The model under review builds one solid part; all positions refer to its coordinate system, in mm. Face numbers are marked on the shaded views. A direction names the side the tool comes from. Give positions to 0.01 mm unless a question says otherwise; leave off trailing zeros. Order: outer loops, then holes, each group sorted by start corner. A loop starts at its lowest first (then second) coordinate and runs counter-clockwise, first axis right, second up.
```python
from build123d import *

# Parameters (mm, degrees)
F0_R     = 32.4890265079
F0_R_2   = 26.7459939795
F1_DEPTH = 50.8
F2_DEPTH = 25.4
F3_W     = 12.6311182976
F3_H     = 77.5911509991
F4_DEPTH = 88.9
F5_DEPTH = 1.7660884187


with BuildPart() as f1:
    # F0 (on Top) → F1 (new body)
    with BuildSketch(Plane.XY):
        Circle(F0_R)
        Circle(F0_R_2, mode=Mode.SUBTRACT)
    extrude(amount=F1_DEPTH)

    # F2 (add): a face of the model
    f2_faces = [f1.faces().sort_by_distance(p)[0] for p in [
        (-31.5700980696, 0, 0),
    ]]
    extrude(f2_faces, amount=F2_DEPTH)

    # F3 (on Front) → F4 (join)
    with BuildSketch(Plane.XZ):
        with Locations((0, 11.1875087023)):
            Rectangle(F3_W, F3_H)
    extrude(amount=F4_DEPTH)

    # F5 (add): a face of the model
    f5_faces = [f1.faces().sort_by_distance(p)[0] for p in [
        (0, -60.5913176327, 49.9830842018),
    ]]
    extrude(f5_faces, amount=F5_DEPTH)


solid = f1.part
```
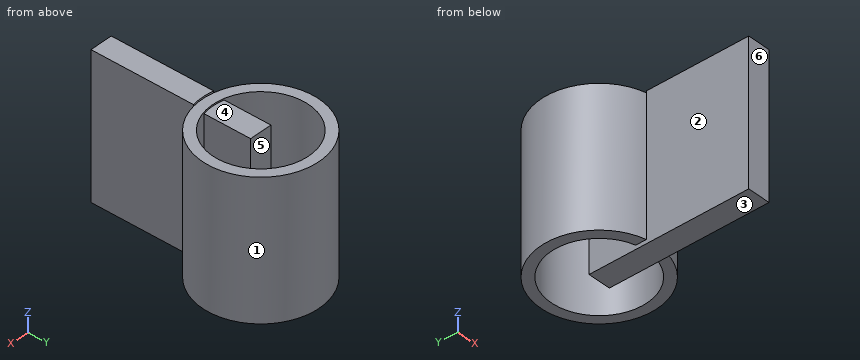
1. Take a section at B-B (y = 16). Write out the cut boundary in (x, z), and give its area (3 significant figures).
2. Draft analysis for pull direction Y (two halves, no side actions). For the marked faces 1, 2, 3 and 4, state which applies: pulls with the +Y half, pulls with the -Y half, needs draft (parallel to the pull), parting line crosses it, or undercut.
3. For the marked faces 5 and 6, list the 3-axis set-ups (+Z, -Z, +X, -X, +Y, -Y) from which the entire face can be reached by the end or side of a thin tool; tool diameter is ignored.
4. Take a section at D-D (z = 39.5). Write out the cut boundary in (x, y), and give its area (3 significant figures).
5. To check wall thickness, follow line 1 (X direction, y = -7, z = 12); line 2 (Y direction, x = 0, z = 20); line 3 (X direction, y = -62, z = -13.5). State the ranges of each line that lie inside material, in increasing order.
6. Insertion check: pin 1 (1 mm diameter, centred on x = 13, z = 14.5, fed in from +Y); pin 2 (10 mm diameter, centred on x = -10, y = -7, fed in from +Z); pin 3 (2 mm diameter, centred on x = -6, z = 19.5, fed in from +Y). Each pin has a flat end and moves straight along its axis. Give the tip position at first contact, or say it passes through.
7. Take a section at A-A (x = 0). Write out the cut boundary in (y, z), and give its area (3 significant figures).
8. Take a section at C-C (y = -10.5). Write out the cut boundary in (x, z), and give its area (3 significant figures).
Answer:
1. outline: (-28.28, -25.4) - (-21.43, -25.4) - (-21.43, 50.8) - (-28.28, 50.8) - close; (21.43, -25.4) - (28.28, -25.4) - (28.28, 50.8) - (21.43, 50.8) - close
1. area: 1,040 mm2
2. face 1: parting line crosses it
2. face 2: undercut
2. face 3: needs draft
2. face 4: undercut
3. face 5: +Z, -Z
3. face 6: +Z, -Z, +X, -X, -Y
4. outline: (-6.32, -88.9) - (6.32, -88.9) - (6.32, -31.87) arc R32.49 ccw (long way) to (-6.32, -31.87) - close; hole (-6.32, -25.99) - (-6.32, 0) - (6.32, 0) - (6.32, -25.99) arc R26.75 ccw (long way) to start
4. area: 2,120 mm2
5. line 1: x = -31.73 to -25.81, -6.32 to 6.32, 25.81 to 31.73
5. line 2: y = -88.9 to 0, 26.75 to 32.49
5. line 3: x = -6.32 to 6.32
6. pin 1: stops at y = 29.99
6. pin 2: stops at z = 49.98
6. pin 3: stops at y = 32.1
7. outline: (-88.9, -27.61) - (0, -27.61) - (0, 49.98) - (-26.75, 49.98) - (-26.75, 50.8) - (-32.49, 50.8) - (-32.49, 51.75) - (-88.9, 51.75) - close; (26.75, -25.4) - (32.49, -25.4) - (32.49, 50.8) - (26.75, 50.8) - close
7. area: 7,440 mm2
8. outline: (-30.75, -25.4) - (-24.6, -25.4) - (-24.6, 50.8) - (-30.75, 50.8) - close; (-6.32, -27.61) - (6.32, -27.61) - (6.32, 49.98) - (-6.32, 49.98) - close; (24.6, -25.4) - (30.75, -25.4) - (30.75, 50.8) - (24.6, 50.8) - close
8. area: 1,920 mm2
